Check sheet for the modelled part. Datum: model origin and axes. Units: mm. Face numbers are marked on the shaded views. Give positions to 0.01 mm unless a question says otherwise; leave off trailing zeros. Loops run counter-clockwise (first coordinate to the right, second up) from the corner with the lowest first, then second, coordinate; pieces in that order, holes last. Notation, with made-up numbers: M -20.5,-29 L 18.5,-29 A32 ccw 18.5,5 Z; hole C 51.25,-30.5 d1. An arc over 180 degrees is marked long. Use one line per item in the form item = value.
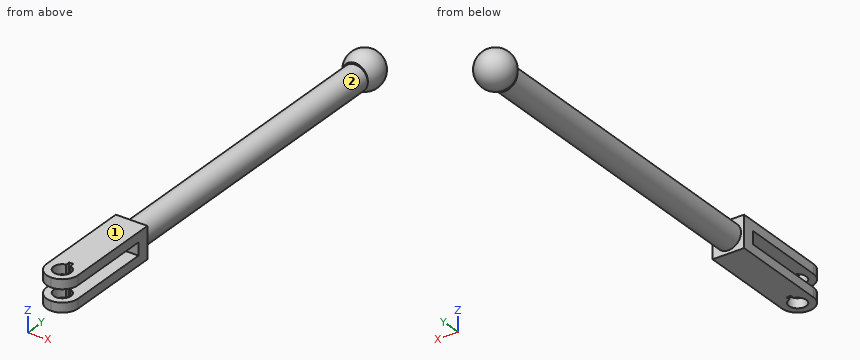
Autodesk Inventor part; units mm, degrees
ref_plane "YZ Plane" through (0, 0, 0) normal (1, 0, 0) x (0, 1, 0)
ref_plane "XZ Plane" through (0, 0, 0) normal (0, 1, 0) x (-1, 0, 0)
ref_plane "XY Plane" through (0, 0, 0) normal (0, 0, 1) x (1, 0, 0)
sketch "Sketch1" plane through (0, 0, 0) normal (1, 0, 0) x (0, 1, 0)
  line L0 (0, 4.5) -> (36, 4.5)
  line L1 (36, 4.5) -> (36, -5.5)
  line L2 (36, -5.5) -> (0, -5.5)
  line L3 (0, -5.5) -> (0, -2.5)
  line L4 (0, -2.5) -> (32, -2.5)
  line L5 (32, -2.5) -> (32, 1.5)
  line L6 (32, 1.5) -> (0, 1.5)
  line L7 (0, 1.5) -> (0, 4.5)
  point P0 (0, 0)
  dimension "d0" = 3
  dimension "d1" = 32
  dimension "d2" = 4
  dimension "d3" = 4
  dimension "d11" = 2.5
  dimension "d12" = 0
extrude "Extrusion1" add sketch "Sketch1" along normal blind 10
sketch "Sketch2" plane through (0, 36, 4.5) normal (0, 1, 0) x (1, 0, 0)
  circle A0 centre (5, 5) radius 4
  line L0 (0, 0) -> (0, 10)
  line L1 (0, 10) -> (10, 10)
  point P0 (0, 4.5)
  dimension "d6" = 8
  dimension "d7" = 5
  dimension "d8" = 5
extrude "Extrusion2" add sketch "Sketch2" along normal blind 100
sketch "Sketch3" plane through (0, 0, 0) normal (0, 0, 1) x (1, 0, 0)
  line L0 (9, 136) -> (1, 136)
  line L1 (1, 136) -> (5, 136)
  line L2 (5, 136) -> (5, 146)
  arc A0 (5, 146) -> (1, 136) centre (5, 140.2) ccw
  point P0 (0, 0)
  dimension "d13" = 10
revolve "Revolution1" add sketch "Sketch3" angle 360 about axis through (5, 136, 0) along (0, 1, 0)
fillet "Fillet1" radius 5 4 edges at (0, 0, -4) (10, 0, -4) (10, 0, 3) (0, 0, 3)
hole "Hole1" at (5, 5, -5.5) direction (0, 0, 1) diameter 5.5 end through all
sketch "Sketch4" plane through (10, 36, -5.5) normal (0, 0, -1) x (-1, 0, 0)
  circle A0 centre (5, -31) radius 2.75
  line L0 (4.325, -28.3341) -> (4.325, -26.9841)
  line L1 (4.325, -26.9841) -> (5.675, -26.9841)
  line L2 (5.675, -26.9841) -> (5.675, -28.3341)
  line L3 (4.325, -28.3341) -> (5.675, -28.3341)
  point P0 (10, -36)
  dimension "d25" = 1.35
  dimension "d26" = 0.675
  dimension "d27" = 1.35
extrude "Extrusion3" cut sketch "Sketch4" against normal through all contours A0 L0 L1 L2
properties part number "EndJoint"
1) Section check B-B (y = 88). Record the cut outline in (x, z), then the cut area to 3 significant figures.
Evaluation:
outline = C 5,-0.5 d8
area = 50.3 mm^2
2) Section check A-A (y = 30). Record the cut outline in (x, z), then the cut area to 3 significant figures.
Evaluation:
outline = M 0,-5.5 L 10,-5.5 L 10,-2.5 L 0,-2.5 Z; M 0,1.5 L 10,1.5 L 10,4.5 L 0,4.5 Z
area = 60.0 mm^2
3) Scan lines: line 1 (X direction, y = 5, z = 2.45); line 2 (Y direction, x = 3.25, z = 3.5); line 3 (Y direction, x = 5, z = -4.85). Record each from-to range of solid material in increasing order.
Evaluation:
line_1 = 0 to 2.25, 7.75 to 10
line_2 = 0.32 to 2.88, 7.12 to 36, 136 to 144.48
line_3 = 0 to 2.25, 9.02 to 36, 137.02 to 143.38
4) Depth check by flat-ended pin: pin 1 Ø1.5 at (y, z) = (8.5, -3.5) entering from +X; pin 2 Ø3 at (x, y) = (4, 24) entering from -Z; pin 3 Ø4.5 at (x, z) = (4.5, 0) entering from -Y; pin 4 Ø6 at (x, z) = (8, -2.5) entering from +Y. Enter the tip coordinate at first touch or a pass-through.
Evaluation:
pin_1 = 10
pin_2 = -5.5
pin_3 = 0
pin_4 = 145.93
5) Release check for a two-part mould opening along Y. For the marked faces 1 and 2 record: pulls with the +Y half, pulls with the -Y half, needs draft (parallel to the pull), parting line crosses it, or undercut.
Evaluation:
face_1 = needs draft
face_2 = undercut
